from build123d import *

# Parameters (mm, degrees)
SKETCH_1_W                  = 30
SKETCH_1_H                  = 35
EXTRUDE_1_DEPTH             = 10
CHAMFER_1_SIZE              = 0.5
SKETCH_7_W                  = 31.194113832
SKETCH_7_H                  = 36.870983812
CUT_EXTRUDE_4_DEPTH         = 1
SKETCH_8_R                  = 5
EXTRUDE_2_DEPTH             = 16
SKETCH_9_R                  = 8.5
SKETCH_9_R_2                = 5
EXTRUDE_3_DEPTH             = 4
SKETCH_10_R                 = 7.5
SKETCH_10_R_2               = 5
EXTRUDE_4_DEPTH             = 2
SKETCH_11_R                 = 5
SKETCH_11_R_2               = 4.75
CUT_EXTRUDE_5_DEPTH         = 1
HOLE_WIZARD_M3_1_AT_2_COUNT = 2
HOLE_WIZARD_M3_1_AT_2_PITCH = 22
SKETCH_13_W                 = 30
SKETCH_13_H                 = 1
CUT_EXTRUDE_6_DEPTH         = 41.926763859


with BuildPart() as part:
    # 草图1 → 凸台-拉伸1 (new body)
    with BuildSketch(Plane(origin=(0, 0, 0), x_dir=(1, 0, 0), z_dir=(0, 1, 0))):
        Rectangle(SKETCH_1_W, SKETCH_1_H)
    extrude(amount=EXTRUDE_1_DEPTH)

    # 倒角1
    chamfer_1_edges = [part.edges().sort_by_distance(p)[0] for p in [
        (15, 5, 17.5),
        (-15, 5, 17.5),
        (-15, 5, -17.5),
        (15, 5, -17.5),
    ]]
    chamfer(chamfer_1_edges, length=CHAMFER_1_SIZE)

    # 草图7 → 切除-拉伸4 (cut)
    with BuildSketch(Plane.XZ):
        Rectangle(SKETCH_7_W, SKETCH_7_H)
    extrude(amount=-CUT_EXTRUDE_4_DEPTH, mode=Mode.SUBTRACT)

    # 草图8 → 凸台-拉伸2 (add)
    with BuildSketch(Plane.XZ.offset(-1)):
        with Locations(Location((0, 0, 0), (0, 0, 270))):
            Circle(SKETCH_8_R)
    extrude(amount=EXTRUDE_2_DEPTH)

    # 草图9 → 凸台-拉伸3 (add)
    with BuildSketch(Plane.XZ.offset(-1)):
        with Locations(Location((0, 0, 0), (0, 0, 270))):
            Circle(SKETCH_9_R)
        with Locations(Location((0, 0, 0), (0, 0, 270))):
            Circle(SKETCH_9_R_2, mode=Mode.SUBTRACT)
    extrude(amount=EXTRUDE_3_DEPTH)

    # 草图10 → 凸台-拉伸4 (add)
    with BuildSketch(Plane.XZ.offset(3)):
        with Locations(Location((0, 0, 0), (0, 0, 270))):
            Circle(SKETCH_10_R)
        with Locations(Location((0, 0, 0), (0, 0, 270))):
            Circle(SKETCH_10_R_2, mode=Mode.SUBTRACT)
    extrude(amount=EXTRUDE_4_DEPTH)

    # 草图11 → 切除-拉伸5 (cut)
    with BuildSketch(Plane(origin=(0, -13, 0), x_dir=(-1, 0, 0), z_dir=(0, -1, 0))):
        with Locations(Location((0, 0, 0), (0, 0, 90))):
            Circle(SKETCH_11_R)
        with Locations(Location((0, 0, 0), (0, 0, 90))):
            Circle(SKETCH_11_R_2, mode=Mode.SUBTRACT)
    extrude(amount=CUT_EXTRUDE_5_DEPTH, mode=Mode.SUBTRACT)

    # 草图12 → M3 螺纹孔1 (revolve, cut)
    with BuildSketch(Plane(origin=(11, 5, 17.5), x_dir=(0, -1, 0), z_dir=(1, 0, 0))):
        Polygon((0, 0), (0, 8.751075774), (1.25, 8), (1.25, 0), align=None)
    hole_wizard_m3_1 = revolve(axis=Axis((11, 5, 23.85), (0, 0, -1)), mode=Mode.SUBTRACT)

    # M3 螺纹孔1 at 2: M3 螺纹孔1 ×2
    with Locations(*[(-i * HOLE_WIZARD_M3_1_AT_2_PITCH, 0, 0) for i in range(1, HOLE_WIZARD_M3_1_AT_2_COUNT)]):
        add(hole_wizard_m3_1, mode=Mode.SUBTRACT)

    # 镜向1: M3 螺纹孔1 across plane
    add(hole_wizard_m3_1.mirror(Plane.XY), mode=Mode.SUBTRACT)

    # 镜向1 copy 1 sketch → 镜向1 copy 1 (revolve, cut)
    with BuildSketch(Plane(origin=(-11, 5, -17.5), x_dir=(0, -1, 0), z_dir=(1, 0, 0))):
        Polygon((0, 0), (0, -8.751075774), (1.25, -8), (1.25, 0), align=None)
    revolve(axis=Axis((-11, 5, -23.85), (0, 0, -1)), mode=Mode.SUBTRACT)

    # 草图13 → 切除-拉伸6 (cut, through all)
    with BuildSketch(Plane(origin=(0, 0, -17.5), x_dir=(-1, 0, 0), z_dir=(0, 0, -1))):
        with Locations((0, 9.5)):
            Rectangle(SKETCH_13_W, SKETCH_13_H)
    extrude(amount=-CUT_EXTRUDE_6_DEPTH, mode=Mode.SUBTRACT)


solid = part.part
Here's how the part is built. I have some questions about the finished solid (model axes, mm). A direction names the side the tool comes from. Round coordinates to 2 decimals unless told otherwise and drop trailing zeros. Write each loop counter-clockwise with the first axis right and the second up, starting at its lowest first coordinate (ties: lowest second). Pieces come first, ordered by that corner, then holes. Notation, with made-up numbers: (7.25, -4) -> (11.25, -4) arc R25 ccw to (11.25, 11) -> close; hole circle Ø11 at (32.25, 55.5). An arc over 180 degrees is marked (long way). One line per item, written item: value.
1) For faces 5 (the face through (-2.89, -13.49, 3.77)), 6 (the face through (-8, -3, 0)), 7 (the face through (9.76, 5.16, 13.56)), which set-ups out of +Z, -Z, +X, -X, +Y, -Y let a thin tool reach every point of the face, with its end or its side?
Filled sheet:
face 5: none
face 6: -Y
face 7: +Z
2) If I drill on line 1 (X direction, y = 5, z = 14); line 2 (Y direction, x = 11, z = 12); line 3 (Y direction, x = 11.25, z = -3), over which ranges is the centre line in solid material (lowest first)? Write a range as [from, to].
Filled sheet:
line 1: x = [-15, -12.25], [-9.75, 9.75], [12.25, 15]
line 2: y = [1, 3.75], [6.25, 9]
line 3: y = [1, 9]
3) Suppose I cut it at B-B on x = 0. List the corners of the cut face in (y, z) for me, plus the area to 4 significant figures.
Filled sheet:
outline: (-15, -5) -> (-14, -5) -> (-14, -4.75) -> (-13, -4.75) -> (-13, -5) -> (-5, -5) -> (-5, -7.5) -> (-3, -7.5) -> (-3, -8.5) -> (1, -8.5) -> (1, -17.5) -> (9, -17.5) -> (9, 17.5) -> (1, 17.5) -> (1, 8.5) -> (-3, 8.5) -> (-3, 7.5) -> (-5, 7.5) -> (-5, 5) -> (-13, 5) -> (-13, 4.75) -> (-14, 4.75) -> (-14, 5) -> (-15, 5) -> close
area: 477.5 mm2
4) I'm going to push flat-ended pins straight in: pin 1 Ø1.5 at (y, z) = (-7, 3) entering from +X; pin 2 Ø8 at (y, z) = (-5.5, -2.5) entering from +X; pin 3 Ø2 at (x, y) = (11, 5) entering from +Z. Where does each tip first touch, or does it pass through?
Filled sheet:
pin 1: stops at x = 4.47
pin 2: stops at x = 8.5
pin 3: stops at z = 9.35
5) Suppose I cut it at D-D on y = -3.5. List the corners of the cut face in (x, z) for me, plus the area to 3 significant figures.
Filled sheet:
outline: circle Ø15 at (0, 0)
area: 177 mm2
6) Suppose I cut it at C-C on z = 0. List the corners of the cut face in (x, y) for me, plus the area to 4 significant figures.
Filled sheet:
outline: (-15, 1) -> (-8.5, 1) -> (-8.5, -3) -> (-7.5, -3) -> (-7.5, -5) -> (-5, -5) -> (-5, -13) -> (-4.75, -13) -> (-4.75, -14) -> (-5, -14) -> (-5, -15) -> (5, -15) -> (5, -14) -> (4.75, -14) -> (4.75, -13) -> (5, -13) -> (5, -5) -> (7.5, -5) -> (7.5, -3) -> (8.5, -3) -> (8.5, 1) -> (15, 1) -> (15, 9) -> (-15, 9) -> close
area: 437.5 mm2
7) Suppose I cut it at A-A on z = 11.5. List the corners of the cut face in (x, y) for me.
Filled sheet:
outline: (-15, 1) -> (15, 1) -> (15, 9) -> (-15, 9) -> close; hole circle Ø2.5 at (-11, 5); hole circle Ø2.5 at (11, 5)
8) We'd pull the mould along Y, two halves only. Please class faces 1 (the face through (-15, 5, 0)), 2 (the face through (9.76, 5.16, -13.56)), 3 (the face through (10.99, 5.22, -8.88)), 4 (the face through (0, 9, 0)): released by +Y, released by -Y, zero draft, split by the parting line, or undercut.
Filled sheet:
face 1: zero draft
face 2: undercut
face 3: undercut
face 4: released by +Y
